The model under review builds one solid part; all positions refer to its coordinate system, in mm. A direction names the side the tool comes from. Round coordinates to 2 decimals unless told otherwise and drop trailing zeros. Loops run counter-clockwise (first coordinate to the right, second up) from the corner with the lowest first, then second, coordinate; pieces in that order, holes last. Notation, with made-up numbers: M 22,-32 L 34,-32 A26 cw 34,-17 Z; hole C -26.5,38.5 d8. An arc over 180 degrees is marked long. Answer as a JSON object with one key per item and string values. Group by question number.
Item 1: The part is to be moulded in two halves that separate along X. For faces 5 (the face through (92, 37, -70)), 6 (the face through (-11, 38, -55)), 7 (the face through (67, 17, -72)), 8 (the face through (-6, 38, -70)), say which applies: +X half, -X half, draft (parallel to the pull), parting line (faces both ways), or undercut.
Item 2: Consider section C-C (z = -79). Give the boundary of the cut face in (x, y).
Item 3: Insertion check: P1, Ø3, axis at y = 17, z = -69.5, coming from the -X side; P2, Ø3, axis at y = 49, z = -64, coming from the +X side; P3, Ø1.8, axis at x = 50.5, y = 15.5, coming from the -Z side; P4, Ø4, axis at x = 97, y = 49.25, coming from the +Z side. Each pin has a flat end and moves straight along its axis. Give the tip position at first contact, or say it passes through.
Item 4: Consider section B-B (y = 25.75). Give the boundary of the cut face in (x, z).
Item 5: To check wall thickness, follow line 1 (X direction, y = 18.6, z = -72.5); line 2 (X direction, y = 49, z = -47); line 3 (Z direction, x = 5.5, y = 15.85). State the ranges of each line that lie inside material, in increasing order.
Item 6: Tool access review of faces 1 (the face through (102, 38, -50)), 2 (the face through (86, 38, -67)), 3 (the face through (97, 38, -55)), 4 (the face through (17, 58, -72)): name each direction out of +Z, -Z, +X, -X, +Y, -Y from which nothing blocks a thin tool from reaching the whole face with its end or side.
Item 7: Consider section D-D (y = 57.5). Give the boundary of the cut face in (x, z), and give its area (3 significant figures).
Item 8: Consider section A-A (x = 5.5). Give the boundary of the cut face in (y, z).
```python
from build123d import *

# Parameters (mm, degrees)
BOSS_EXTRUDE2_DEPTH    = 75
SKETCH3_W              = 20
SKETCH3_H              = 10
BOSS_EXTRUDE3_DEPTH    = 75
SKETCH4_W              = 50
SKETCH4_H              = 25
CUT_EXTRUDE1_DEPTH     = 75
SKETCH5_W              = 50
SKETCH5_H              = 28
CUT_EXTRUDE2_DEPTH     = 75
SKETCH6_W              = 19
SKETCH6_H              = 35
CUT_EXTRUDE3_DEPTH     = 25
CUT_EXTRUDE4_DEPTH     = 14
CUT_EXTRUDE5_DEPTH     = 14
SKETCH24_W             = 50
SKETCH24_H             = 10
BOSS_EXTRUDE4_DEPTH    = 6
SKETCH25_W             = 50
SKETCH25_H             = 10
BOSS_EXTRUDE5_DEPTH    = 6
CUT_EXTRUDE7_DEPTH     = 143.751532391
SKETCH33_W             = 10
SKETCH33_H             = 10
BOSS_EXTRUDE6_DEPTH    = 47
M4X0_7_TAPPED_HOLE8_D  = 3.3
M4X0_7_TAPPED_HOLE9_D  = 3.3
M4X0_7_TAPPED_HOLE10_D = 3.3
M4X0_7_TAPPED_HOLE11_D = 3.3
BOSS_EXTRUDE7_DEPTH    = 10
BOSS_EXTRUDE8_DEPTH    = 10
M4X0_7_TAPPED_HOLE12_D = 3.3
M4X0_7_TAPPED_HOLE13_D = 3.3


with BuildPart() as part:
    # Sketch2 → Boss-Extrude2 (new body)
    with BuildSketch(Plane(origin=(0, 0, 0), x_dir=(1, 0, 0), z_dir=(0, 1, 0))):
        Polygon((-6, 69), (-6, 0), (-6, -6), (0, -6), (86, -6), (92, -6), (92, 0), (92, 69), (92, 75), (86, 75), (0, 75), (-6, 75), align=None)
    extrude(amount=BOSS_EXTRUDE2_DEPTH)

    # Sketch3 → Boss-Extrude3 (add)
    with BuildSketch(Plane(origin=(0, 0, 0), x_dir=(-1, 0, 0), z_dir=(0, -1, 0))):
        with Locations((-102, -1)):
            Rectangle(SKETCH3_W, SKETCH3_H)
        with Locations((16, -1)):
            Rectangle(SKETCH3_W, SKETCH3_H)
    extrude(amount=-BOSS_EXTRUDE3_DEPTH)

    # Sketch4 → Cut-Extrude1 (cut)
    with BuildSketch(Plane(origin=(0, 0, 0), x_dir=(-1, 0, 0), z_dir=(0, -1, 0))):
        with Locations((-42, 62.5)):
            Rectangle(SKETCH4_W, SKETCH4_H)
    extrude(amount=-CUT_EXTRUDE1_DEPTH, mode=Mode.SUBTRACT)

    # Sketch5 → Cut-Extrude2 (cut)
    with BuildSketch(Plane(origin=(0, 0, 0), x_dir=(-1, 0, 0), z_dir=(0, -1, 0))):
        with Locations((-42, 8)):
            Rectangle(SKETCH5_W, SKETCH5_H)
    extrude(amount=-CUT_EXTRUDE2_DEPTH, mode=Mode.SUBTRACT)

    # Sketch6 → Cut-Extrude3 (cut)
    with BuildSketch(Plane(origin=(0, 0, -75), x_dir=(-1, 0, 0), z_dir=(0, 0, -1))):
        with Locations((-76.5, 37.5)):
            Rectangle(SKETCH6_W, SKETCH6_H)
        Polygon((-67, 55), (-67, 20), (0, 20), (0, 37.5), (0, 55), align=None)
    extrude(amount=-CUT_EXTRUDE3_DEPTH, mode=Mode.SUBTRACT)

    # Sketch7 → Cut-Extrude4 (cut)
    with BuildSketch(Plane(origin=(0, 0, 0), x_dir=(-1, 0, 0), z_dir=(0, -1, 0))):
        Polygon((-112, 4), (-112, -6), (-67, -6), (-67, 22), (-17, 22), (-17, -6), (26, -6), (26, 4), (6, 4), (6, 75), (-17, 75), (-17, 50), (-67, 50), (-67, 75), (-92, 75), (-92, 4), align=None)
    extrude(amount=-CUT_EXTRUDE4_DEPTH, mode=Mode.SUBTRACT)

    # Sketch8 → Cut-Extrude5 (cut)
    with BuildSketch(Plane(origin=(0, 75, 0), x_dir=(1, 0, 0), z_dir=(0, 1, 0))):
        Polygon((-26, 4), (-6, 4), (-6, 75), (17, 75), (17, 50), (67, 50), (67, 75), (92, 75), (92, 4), (112, 4), (112, -6), (67, -6), (67, 22), (17, 22), (17, -6), (-26, -6), align=None)
    extrude(amount=-CUT_EXTRUDE5_DEPTH, mode=Mode.SUBTRACT)

    # Sketch24 → Boss-Extrude4 (add)
    with BuildSketch(Plane(origin=(0, 14, 0), x_dir=(-1, 0, 0), z_dir=(0, -1, 0))):
        with Locations((-42, 55)):
            Rectangle(SKETCH24_W, SKETCH24_H)
    extrude(amount=-BOSS_EXTRUDE4_DEPTH)

    # Sketch25 → Boss-Extrude5 (add)
    with BuildSketch(Plane(origin=(0, 61, 0), x_dir=(1, 0, 0), z_dir=(0, 1, 0))):
        with Locations((42, 55)):
            Rectangle(SKETCH25_W, SKETCH25_H)
    extrude(amount=-BOSS_EXTRUDE5_DEPTH)

    # Sketch31 → Cut-Extrude7 (cut, through all)
    with BuildSketch(Plane(origin=(0, 61, 0), x_dir=(1, 0, 0), z_dir=(0, 1, 0))):
        Polygon((-6, 45), (92, 45), (112, 45), (112, -6), (92, -6), (-6, -6), (-26, -6), (-26, 45), align=None)
    extrude(amount=-CUT_EXTRUDE7_DEPTH, mode=Mode.SUBTRACT)

    # Sketch33 → Boss-Extrude6 (add, through all)
    with BuildSketch(Plane(origin=(0, 61, 0), x_dir=(1, 0, 0), z_dir=(0, 1, 0))):
        with Locations((-11, 50)):
            Rectangle(SKETCH33_W, SKETCH33_H)
        with Locations((97, 50)):
            Rectangle(SKETCH33_W, SKETCH33_H)
    extrude(amount=-BOSS_EXTRUDE6_DEPTH)

    # M4x0.7 Tapped Hole8 (through all)
    with Locations(Plane(origin=(0, 0, -55), x_dir=(-1, 0, 0), z_dir=(0, 0, -1))):
        with Locations((11, 25.75)):
            Hole(M4X0_7_TAPPED_HOLE8_D / 2)

    # M4x0.7 Tapped Hole9 (through all)
    with Locations(Plane(origin=(0, 0, -55), x_dir=(-1, 0, 0), z_dir=(0, 0, -1))):
        with Locations((11, 49.25)):
            Hole(M4X0_7_TAPPED_HOLE9_D / 2)

    # M4x0.7 Tapped Hole10 (through all)
    with Locations(Plane(origin=(0, 0, -55), x_dir=(-1, 0, 0), z_dir=(0, 0, -1))):
        with Locations((-97, 49.25)):
            Hole(M4X0_7_TAPPED_HOLE10_D / 2)

    # M4x0.7 Tapped Hole11 (through all)
    with Locations(Plane(origin=(0, 0, -55), x_dir=(-1, 0, 0), z_dir=(0, 0, -1))):
        with Locations((-97, 25.75)):
            Hole(M4X0_7_TAPPED_HOLE11_D / 2)

    # Sketch44 → Boss-Extrude7 (add)
    with BuildSketch(Plane(origin=(0, 20, -75), x_dir=(-1, 0, 0), z_dir=(0, 0, -1))):
        Polygon((-17, -6), (-17, 0), (0, 0), (0, 35), (-17, 35), (-17, 41), (6, 41), (6, -6), align=None)
    extrude(amount=BOSS_EXTRUDE7_DEPTH)

    # Sketch45 → Boss-Extrude8 (add)
    with BuildSketch(Plane(origin=(0, 0, -75), x_dir=(-1, 0, 0), z_dir=(0, 0, -1))):
        Polygon((-67, 61), (-67, 55), (-86, 55), (-86, 20), (-67, 20), (-67, 14), (-92, 14), (-92, 61), align=None)
    extrude(amount=BOSS_EXTRUDE8_DEPTH)

    # M4x0.7 Tapped Hole12 (through all)
    with Locations(Plane(origin=(0, 61, 0), x_dir=(1, 0, 0), z_dir=(0, 1, 0))):
        with Locations((5.5, 72.5)):
            Hole(M4X0_7_TAPPED_HOLE12_D / 2)

    # M4x0.7 Tapped Hole13 (through all)
    with Locations(Plane(origin=(0, 61, 0), x_dir=(1, 0, 0), z_dir=(0, 1, 0))):
        with Locations((79.5, 72.5)):
            Hole(M4X0_7_TAPPED_HOLE13_D / 2)


solid = part.part
```
Geometry results:
{
 "1": {"face 5": "+X half", "face 6": "draft", "face 7": "undercut", "face 8": "-X half"},
 "2": {"outline": "M -6,14 L 17,14 L 17,20 L 0,20 L 0,55 L 17,55 L 17,61 L -6,61 Z; M 67,14 L 92,14 L 92,61 L 67,61 L 67,55 L 86,55 L 86,20 L 67,20 Z"},
 "3": {"P1": "stops at x = -6", "P2": "stops at x = 92", "P3": "stops at z = -60", "P4": "stops at z = -45"},
 "4": {"outline": "M -16,-55 L -12.65,-55 L -12.65,-45 L -16,-45 Z; M -9.35,-55 L -6,-55 L -6,-85 L 0,-85 L 0,-50 L 86,-50 L 86,-85 L 92,-85 L 92,-55 L 95.35,-55 L 95.35,-45 L -9.35,-45 Z; M 98.65,-55 L 102,-55 L 102,-45 L 98.65,-45 Z"},
 "5": {"line 1": "x = -6 to 3.85, 7.15 to 17, 67 to 77.85, 81.15 to 92", "line 2": "x = -16 to -12.63, -9.37 to 95.37, 98.63 to 102", "line 3": "z = -85 to -74.15, -70.85 to -45"},
 "6": {"face 1": "+Z, -Z, +X, +Y, -Y", "face 2": "-Z", "face 3": "-Z, +X, +Y, -Y", "face 4": "-Z, +Y, -Y"},
 "7": {"outline": "M -16,-55 L -6,-55 L -6,-85 L 17,-85 L 17,-60 L 67,-60 L 67,-85 L 92,-85 L 92,-55 L 102,-55 L 102,-45 L -16,-45 Z; hole C 5.5,-72.5 d3.3; hole C 79.5,-72.5 d3.3", "area": "2,850 mm^2"},
 "8": {"outline": "M 14,-85 L 20,-85 L 20,-74.15 L 14,-74.15 Z; M 14,-70.85 L 20,-70.85 L 20,-50 L 55,-50 L 55,-70.85 L 61,-70.85 L 61,-45 L 14,-45 Z; M 55,-85 L 61,-85 L 61,-74.15 L 55,-74.15 Z"}
}
